```python
from build123d import *

# Parameters (mm, degrees)
F1_DEPTH = 20
F3_D     = 6.6
F3_DEPTH = 43
F3_TIP   = 1.9828400428
F4_R     = 5


with BuildPart() as f1:
    # F0 (on Right) → F1 (new body, symmetric)
    with BuildSketch(Plane.YZ):
        Polygon((0, 0), (0, -0.75), (35, -0.75), (35, 0.75), (0, 0.75), align=None)
    extrude(amount=F1_DEPTH, both=True)

    # F3
    with Locations(Plane.XY.offset(0.75)):
        with Locations((-10.5, 7), (10.5, 7), (10.5, 22), (-10.5, 22)):
            Hole(F3_D / 2, depth=F3_DEPTH)
            with Locations((0, 0, -(F3_DEPTH + F3_TIP / 2))):  # 118° drill point
                Cone(0, F3_D / 2, F3_TIP, mode=Mode.SUBTRACT)

    # F4
    f4_edges = [f1.edges().sort_by_distance(p)[0] for p in [
        (20, 0, 0),
        (-20, 0, 0),
        (20, 35, 0),
        (-20, 35, 0),
    ]]
    fillet(f4_edges, radius=F4_R)


solid = f1.part
```
Work out the finished part from the listing and answer in its coordinate system (mm). Round coordinates to 2 decimals unless told otherwise and drop trailing zeros. Write each loop counter-clockwise with the first axis right and the second up, starting at its lowest first coordinate (ties: lowest second). Pieces come first, ordered by that corner, then holes.
1) A cutting plane is placed at A-A on x = 10.5. Determine the outline of the cut face in (y, z).
2) A flat-ended cylindrical pin translates along its axis: P1, Ø5.5, axis at x = -10.5, y = 22, coming from the +Z side. Find the tip coordinate at first contact, or state that the pin passes through.
3) Determine the mould class of faces 1 (the face through (-19, 2, 0)), 2 (the face through (13.8, 7.1, 0)), 3 (the face through (-20, 17, 0)) for opening direction Y: pulls with the +Y half, pulls with the -Y half, needs draft (parallel to the pull), parting line crosses it, or undercut.
4) A cutting plane is placed at D-D on y = 32. Determine the outline of the cut face in (x, z).
5) A cutting plane is placed at B-B on y = 22. Determine the outline of the cut face in (x, z).
6) A cutting plane is placed at C-C on z = 0.1. Determine the outline of the cut face in (x, y), and give its area (3 significant figures).
7) Consider probe 1 along Y at (x, z) = (10.5, 0); probe 2 along Y at (x, z) = (12, 0.15); probe 3 along X at (y, z) = (19, 0). Determine where each line is inside the solid, lowest interval first.
Entries:
1. outline: (0, -0.75) - (3.7, -0.75) - (3.7, 0.75) - (0, 0.75) - close; (10.3, -0.75) - (18.7, -0.75) - (18.7, 0.75) - (10.3, 0.75) - close; (25.3, -0.75) - (35, -0.75) - (35, 0.75) - (25.3, 0.75) - close
2. P1: passes through
3. face 1: pulls with the -Y half
3. face 2: undercut
3. face 3: needs draft
4. outline: (-19.58, -0.75) - (19.58, -0.75) - (19.58, 0.75) - (-19.58, 0.75) - close
5. outline: (-20, -0.75) - (-13.8, -0.75) - (-13.8, 0.75) - (-20, 0.75) - close; (-7.2, -0.75) - (7.2, -0.75) - (7.2, 0.75) - (-7.2, 0.75) - close; (13.8, -0.75) - (20, -0.75) - (20, 0.75) - (13.8, 0.75) - close
6. outline: (-20, 5) arc R5 ccw to (-15, 0) - (15, 0) arc R5 ccw to (20, 5) - (20, 30) arc R5 ccw to (15, 35) - (-15, 35) arc R5 ccw to (-20, 30) - close; hole circle Ø6.6 at (-10.5, 7); hole circle Ø6.6 at (-10.5, 22); hole circle Ø6.6 at (10.5, 7); hole circle Ø6.6 at (10.5, 22)
6. area: 1,240 mm2
7. probe 1: y = 0 to 3.7, 10.3 to 18.7, 25.3 to 35
7. probe 2: y = 0 to 4.06, 9.94 to 19.06, 24.94 to 35
7. probe 3: x = -20 to -11.87, -9.13 to 9.13, 11.87 to 20
